Design review of the part built by this model. Coordinates are the model's own, in mm. A direction names the side the tool comes from. Round coordinates to 2 decimals unless told otherwise and drop trailing zeros. Loops run counter-clockwise (first coordinate to the right, second up) from the corner with the lowest first, then second, coordinate; pieces in that order, holes last. Notation, with made-up numbers: (-20.5, -20) - (-13.5, -20) arc R19 cw to (-13.5, -4) - close; hole circle Ø11 at (-22, 16). An arc over 180 degrees is marked (long way). Use one line per item in the form item = value. Start each with the question number.
(1) For pin 1 (5 mm diameter, centred on x = 5.5, y = 0.5, fed in from +Z); pin 2 (9 mm diameter, centred on x = 5, z = 26, fed in from -Y), all flat-tipped, find the tip position at first contact; note any pin that passes through.
(2) Wall thickness on probe 1 along X at (y, z) = (2.25, 2.5); probe 2 along X at (y, z) = (0.25, 26); probe 3 along Z at (x, y) = (-0.25, -3.75): over which ranges is each line inside the solid? List them lowest first. Write a range as [from, to].
(3) We need section B-B, the plane z = 19.5. Write out the cut boundary in (x, y), then the cut area to 3 significant figures.
(4) Machinability: for faces 4 (the cylindrical face through (-3.4, 4.43, 10.27)), 5 (the cylindrical face through (2.74, 0.06, 29.49)), 6 (the cylindrical face through (-3.4, -4.43, 10.27)), 7 (the cylindrical face through (13.4, 4.43, 10.56)), 8 (the flat face through (5, 0, 16)), which of the approach directions +Z, -Z, +X, -X, +Y, -Y give a long, thin tool a straight path to every point of the face, cutting with its end or side? Answer none if there is none.
(5) We need section C-C, the plane y = -2.5. Write out the cut boundary in (x, z), then the cut area to 3 significant figures.
(6) The part is to be moulded in two halves that separate along X. For faces 1 (the flat face through (10, 0, 8)), 2 (the cylindrical face through (-2.393, -0.07, 27.263)), 3 (the flat face through (14, 0, 10)), say which applies: released by +X, released by -X, zero draft, split by the parting line, or undercut.
(7) We need section D-D, the plane x = 5. Write out the cut boundary in (y, z), then the cut area to 3 significant figures.
(8) We need section A-A, the plane z = 26. Write out the cut boundary in (x, y), then the cut area to 3 significant figures.
from build123d import *

# Parameters (mm, degrees)
F1_DEPTH    = 5
F2_R        = 7.5
F2_R_2      = 4
F3_DEPTH    = 5
F4_W        = 4
F4_H        = 10
F5_DEPTH    = 5.7
F6_T1_DEPTH = 10
F6_T3_DEPTH = 30.1640895286
F6_T5_DEPTH = 15.0401716993
F7_R        = 2
F8_T2_ANGLE = 359.64
F8_T4_ANGLE = 359.64


# Not quite as in the source:
# - a fillet or chamfer that OpenCascade refuses, or shapes differently, is made with other operations: its cross-section is extruded or revolved along the edge and cut away or added


with BuildPart() as f1:
    # F0 (on Front) → F1 (new body, symmetric)
    with BuildSketch(Plane.XZ):
        Polygon((-4, 0), (0, 0), (0, 16), (10, 16), (10, 0), (14, 0), (14, 20), (-4, 20), align=None)
    extrude(amount=F1_DEPTH, both=True)

    # F2 (on Front) → F3 (join, symmetric)
    with BuildSketch(Plane.XZ):
        with Locations((5, 26)):
            Circle(F2_R)
        with Locations((5, 26)):
            Circle(F2_R_2, mode=Mode.SUBTRACT)
    extrude(amount=F3_DEPTH, both=True)

    # F4 (on Front) → F5 (cut, symmetric)
    with BuildSketch(Plane.XZ):
        with Locations((5, 31.8401088891)):
            Rectangle(F4_W, F4_H)
    extrude(amount=F5_DEPTH, both=True, mode=Mode.SUBTRACT)

    # F6: fillet of radius 2 on 6 edges, made by hand

    # F6_s2 → F6_t1 (join)
    with BuildSketch(Plane.XZ.offset(-5)):
        with BuildLine():
            ThreePointArc((-3.6168439698, 20), (-1.930989509, 20.9239448263), (-1.8027715551, 22.8421052632))
            ThreePointArc((-1.8027715551, 22.8421052632), (-0.8273108539, 21.2785120765), (0.5, 20))
            Line((0.5, 20), (-3.6168439698, 20))
        make_face()
        with BuildLine():
            ThreePointArc((11.8027715551, 22.8421052632), (11.930989509, 20.9239448263), (13.6168439698, 20))
            Line((13.6168439698, 20), (9.5, 20))
            ThreePointArc((9.5, 20), (10.8273108539, 21.2785120765), (11.8027715551, 22.8421052632))
        make_face()
    extrude(amount=F6_T1_DEPTH)

    # F6_s4 → F6_t3 (cut)
    with BuildSketch(Plane.XZ.offset(-15.0820447643)):
        with BuildLine():
            ThreePointArc((10.4545454545, 31.1476143877), (8.2614510541, 31.6335579722), (7, 29.7749172176))
            Line((7, 29.7749172176), (7, 33.2284161474))
            ThreePointArc((7, 33.2284161474), (8.869753994, 32.4245625552), (10.4545454545, 31.1476143877))
        make_face()
        with BuildLine():
            ThreePointArc((3, 29.7749172176), (1.7385489459, 31.6335579722), (-0.4545454545, 31.1476143877))
            ThreePointArc((-0.4545454545, 31.1476143877), (1.130246006, 32.4245625552), (3, 33.2284161474))
            Line((3, 33.2284161474), (3, 29.7749172176))
        make_face()
    extrude(amount=F6_T3_DEPTH, mode=Mode.SUBTRACT)

    # F6_s6 → F6_t5 (cut)
    with BuildSketch(Plane.XZ.offset(-7.5200858497)):
        with BuildLine():
            ThreePointArc((7, 30.472135955), (7.1742581416, 29.6556393741), (7.6666666667, 28.98142397))
            ThreePointArc((7.6666666667, 28.98142397), (7.3457810792, 29.2399554207), (7, 29.4641016151))
            Line((7, 29.4641016151), (7, 30.472135955))
        make_face()
        with BuildLine():
            ThreePointArc((2.3333333333, 28.98142397), (2.8257418584, 29.6556393741), (3, 30.472135955))
            Line((3, 30.472135955), (3, 29.4641016151))
            ThreePointArc((3, 29.4641016151), (2.6542189208, 29.2399554207), (2.3333333333, 28.98142397))
        make_face()
    extrude(amount=F6_T5_DEPTH, mode=Mode.SUBTRACT)

    # F7
    f7_edges = [f1.edges().sort_by_distance(p)[0] for p in [
        (-4, -5, 10),
        (14, -5, 10),
        (14, 5, 10),
        (-4, 5, 10),
    ]]
    fillet(f7_edges, radius=F7_R)

    # F8: fillet of radius 2 on 2 edges, made by hand

    # F8_s1 → F8_t2 (revolve, cut)
    with BuildSketch(Plane(origin=(4.9182697806, 0, -0.015451251), x_dir=(0, 1, 0), z_dir=(-0.9999950652, 0, 0.0031415875))):
        with BuildLine():
            ThreePointArc((-5, -32.0155796327), (-4.4142135624, -30.6013660703), (-3, -30.0155796327))
            Line((-3, -30.0155796327), (-5, -30.0155796327))
            Line((-5, -30.0155796327), (-5, -32.0155796327))
        make_face()
    revolve(axis=Axis((5, -5, 26), (0, 1, 0)), revolution_arc=F8_T2_ANGLE, mode=Mode.SUBTRACT)

    # F8_s3 → F8_t4 (revolve, cut)
    with BuildSketch(Plane(origin=(5.0816315237, 0, 0.0159644688), x_dir=(0, 1, 0), z_dir=(0.9999950652, 0, 0.0031415875))):
        with BuildLine():
            ThreePointArc((5, 31.9841637578), (4.4142135624, 30.5699501954), (3, 29.9841637578))
            Line((3, 29.9841637578), (5, 29.9841637578))
            Line((5, 29.9841637578), (5, 31.9841637578))
        make_face()
    revolve(axis=Axis((5, 5, 26), (0, -1, 0)), revolution_arc=F8_T4_ANGLE, mode=Mode.SUBTRACT)


solid = f1.part
Data:
q1.pin_1 = 31.51
q1.pin_2 = -4.32
q2.probe_1 = [-4, 0], [10, 14]
q2.probe_2 = [-2.5, 1], [9, 12.5]
q2.probe_3 = [0, 31.34]
q3.outline = (-4, -3) arc R2 ccw to (-2, -5) - (12, -5) arc R2 ccw to (14, -3) - (14, 3) arc R2 ccw to (12, 5) - (-2, 5) arc R2 ccw to (-4, 3) - close
q3.area = 177 mm^2
q4.face_4 = -Z, -X, +Y
q4.face_5 = +Y, -Y
q4.face_6 = -Z, -X, -Y
q4.face_7 = -Z, +X, +Y
q4.face_8 = -Z, +Y, -Y
q5.outline = (-4, 0) - (0, 0) - (0, 16) - (10, 16) - (10, 0) - (14, 0) - (14, 20) - (13.62, 20) arc R2 cw to (11.8, 22.84) arc R7.5 ccw to (10.45, 31.15) arc R2 ccw to (7.03, 30.12) arc R2 ccw to (7.67, 28.98) arc R4 cw (long way) to (2.33, 28.98) arc R2 ccw to (2.97, 30.12) arc R2 ccw to (-0.45, 31.15) arc R7.5 ccw to (-1.8, 22.84) arc R2 cw to (-3.62, 20) - (-4, 20) - close
q5.area = 302 mm^2
q6.face_1 = undercut
q6.face_2 = released by -X
q6.face_3 = released by +X
q7.outline = (-5, 16) - (5, 16) - (5, 20) arc R2 ccw to (3, 22) - (-3, 22) arc R2 ccw to (-5, 20) - close
q7.area = 58.3 mm^2
q8.outline = (-2.5, -5) - (-1, -5) arc R2 ccw to (1, -3) - (1, 3) arc R2 ccw to (-1, 5) - (-2.5, 5) - close; (9, -3) arc R2 ccw to (11, -5) - (12.5, -5) - (12.5, 5) - (11, 5) arc R2 ccw to (9, 3) - close
q8.area = 66.6 mm^2
